Here's how the part is built. I have some questions about the finished solid (model axes, mm). Face numbers are marked on the shaded views. Coordinates: 2 decimals unless noted, no trailing zeros. Write each loop counter-clockwise with the first axis right and the second up, starting at its lowest first coordinate (ties: lowest second). Pieces come first, ordered by that corner, then holes. Notation, with made-up numbers: (34, 45) -> (71, 45) arc R5 cw to (71, 52) -> close; hole circle Ø2 at (-6, 17.5). An arc over 180 degrees is marked (long way). Put each result on its own line as item: value. Start each with the question number.
Item 1: For pin 1 (0.6 mm diameter, centred on x = -4.5, y = -1.5, fed in from +Z); pin 2 (2.5 mm diameter, centred on x = 3, z = 3, fed in from +Y), each with a flat end and sliding along its axis, tell me the tip position at first contact or that it passes through.
Item 2: I want a section at B-B, the plane z = 3. List the corners of the cut face in (x, y) for me.
Item 3: If we mould it in two halves opening along Z, with no side actions, what happens to the marked faces 1, 2 and 3? For each: released by +Z, released by -Z, zero draft, split by the parting line, or undercut.
Item 4: I want a section at C-C, the plane y = -1.7. List the corners of the cut face in (x, z) for me, then the cut area to 3 significant figures.
Item 5: I need wall thicknesses on line 1 (Z direction, x = -3, y = -0.45); line 2 (Z direction, x = 1.75, y = -1.5); line 3 (Z direction, x = -4.25, y = -0.55). Which ranges of each line are inside material? Lowest first, please. Write a range as [from, to].
Item 6: I want a section at A-A, the plane x = 3. List the corners of the cut face in (y, z) for me, then the cut area to 3 significant figures.
Item 7: I want a section at D-D, the plane z = 8. List the corners of the cut face in (x, y) for me.
from build123d import *

# Parameters (mm, degrees)
F0_W      = 15
F0_H      = 15
F1_DEPTH  = 2
F2_R      = 1.5
F3_DEPTH  = 25
F4_W      = 9
F4_H      = 2
F5_DEPTH  = 6
F6_R      = 1.5
F7_DEPTH  = 25
F8_R      = 1.5
F9_W      = 15
F9_H      = 2
F10_DEPTH = 1


with BuildPart() as f1:
    # F0 (on Front) → F1 (new body)
    with BuildSketch(Plane.XZ):
        Rectangle(F0_W, F0_H)
    extrude(amount=F1_DEPTH)

    # F2 (on face) → F3 (cut)
    with BuildSketch(Plane.XZ.offset(2)):
        with Locations((3, 3)):
            Circle(F2_R)
        with Locations((-3, 3)):
            Circle(F2_R)
        with Locations((-3, -3)):
            Circle(F2_R)
        with Locations((3, -3)):
            Circle(F2_R)
    extrude(amount=-F3_DEPTH, mode=Mode.SUBTRACT)

    # F4 (on face) → F5 (join)
    with BuildSketch(Plane.XY.offset(7.5)):
        with Locations((3, -1)):
            Rectangle(F4_W, F4_H)
    extrude(amount=F5_DEPTH)

    # F6 (on face) → F7 (cut)
    with BuildSketch(Plane.XZ.offset(2)):
        with Locations((3, 9)):
            Circle(F6_R)
    extrude(amount=-F7_DEPTH, mode=Mode.SUBTRACT)

    # F8
    f8_edges = [f1.edges().sort_by_distance(p)[0] for p in [
        (7.5, -1, 13.5),
        (-1.5, -1, 13.5),
        (-1.5, -1, 7.5),
    ]]
    fillet(f8_edges, radius=F8_R)

    # F9 (on face) → F10 (join)
    with BuildSketch(Plane(origin=(0, 0, -7.5), x_dir=(1, 0, 0), z_dir=(0, 0, -1))):
        with Locations((0, 1)):
            Rectangle(F9_W, F9_H)
    extrude(amount=F10_DEPTH)


solid = f1.part
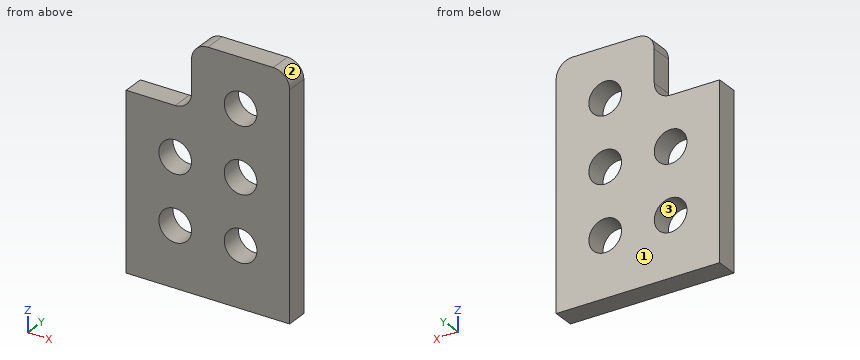
Calculated:
1. pin 1: stops at z = 7.5
1. pin 2: passes through
2. outline: (-7.5, -2) -> (-4.5, -2) -> (-4.5, 0) -> (-7.5, 0) -> close; (-1.5, -2) -> (1.5, -2) -> (1.5, 0) -> (-1.5, 0) -> close; (4.5, -2) -> (7.5, -2) -> (7.5, 0) -> (4.5, 0) -> close
3. face 1: zero draft
3. face 2: released by +Z
3. face 3: undercut
4. outline: (-7.5, -8.5) -> (7.5, -8.5) -> (7.5, 12) arc R1.5 ccw to (6, 13.5) -> (0, 13.5) arc R1.5 ccw to (-1.5, 12) -> (-1.5, 9) arc R1.5 cw to (-3, 7.5) -> (-7.5, 7.5) -> close; hole circle Ø3 at (-3, -3); hole circle Ø3 at (-3, 3); hole circle Ø3 at (3, -3); hole circle Ø3 at (3, 3); hole circle Ø3 at (3, 9)
4. area: 258 mm2
5. line 1: z = [-8.5, -4.5], [-1.5, 1.5], [4.5, 7.5]
5. line 2: z = [-8.5, -3.83], [-2.17, 2.17], [3.83, 8.17], [9.83, 13.5]
5. line 3: z = [-8.5, -3.83], [-2.17, 2.17], [3.83, 7.5]
6. outline: (-2, -8.5) -> (0, -8.5) -> (0, -4.5) -> (-2, -4.5) -> close; (-2, -1.5) -> (0, -1.5) -> (0, 1.5) -> (-2, 1.5) -> close; (-2, 4.5) -> (0, 4.5) -> (0, 7.5) -> (-2, 7.5) -> close; (-2, 10.5) -> (0, 10.5) -> (0, 13.5) -> (-2, 13.5) -> close
6. area: 26.0 mm2
7. outline: (-1.88, -2) -> (1.88, -2) -> (1.88, 0) -> (-1.88, 0) -> close; (4.12, -2) -> (7.5, -2) -> (7.5, 0) -> (4.12, 0) -> close
